Part model, mm, in its own coordinate system. Coordinates: 2 decimals unless noted, no trailing zeros. Loops run counter-clockwise (first coordinate to the right, second up) from the corner with the lowest first, then second, coordinate; pieces in that order, holes last. Notation, with made-up numbers: (-2, -29.75) -> (3, -29.75) arc R8 ccw to (3, -16.75) -> close; hole circle Ø2 at (-30, 59). An arc over 180 degrees is marked (long way). Use one line per item in the form item = value. Start each with the question number.
(1) Mould opens along Z. For faces 1 (the flat face through (0, 0, -9.525)), 2 (the flat face through (0, -4.762, 0)), 3 (the cylindrical face through (-10.349, -0.062, 1.584)) say: +Z half, -Z half, draft (parallel to the pull), parting line (faces both ways), or undercut.
(2) Band-saw the part on B-B on y = 3.5. Give the cut face in (x, z) (1 decimal), then the cut area to 3 significant figures.
(3) Drill centre lines: L1, parallel to X at y = -3, z = 0.75; L2, parallel to X at y = 1, z = -1; L3, parallel to Z at x = 1.75, y = -4.5. Where is each one in solid material? Low to high. Write a range as [from, to].
(4) Band-saw the part on A-A on z = 0. Give the cut face in (x, y) (1 decimal), then the cut area to 3 significant figures.
Autodesk Inventor part; units mm, degrees
ref_plane "YZ Plane" through (0, 0, 0) normal (1, 0, 0) x (0, 1, 0)
ref_plane "XZ Plane" through (0, 0, 0) normal (0, 1, 0) x (-1, 0, 0)
ref_plane "XY Plane" through (0, 0, 0) normal (0, 0, 1) x (1, 0, 0)
sketch "Sketch1" plane through (0, 0, 0) normal (0, 1, 0) x (-1, 0, 0)
  line L0 (-12.7, -9.525) -> (12.7, -9.525)
  line L1 (12.7, -9.525) -> (12.7, 9.525)
  line L2 (12.7, 9.525) -> (-12.7, 9.525)
  line L3 (-12.7, 9.525) -> (-12.7, -9.525)
  line L4 (-12.7, -9.525) -> (12.7, 9.525) construction
  line L5 (12.7, -9.525) -> (-12.7, 9.525) construction
  circle A0 centre (9.525, 0) radius 1.7859
  circle A1 centre (-9.525, 0) radius 1.7859
  point P0 (0, 0)
  dimension "d0" = 25.4
  dimension "d1" = 19.05
  dimension "d2" = 3.5719
  dimension "d3" = 3.5719
  dimension "d4" = 19.05
  dimension "d5" = 3.175
  dimension "d6" = 3.175
  dimension "d7" = 5.715
extrude "Extrusion1" add sketch "Sketch1" along normal mid plane 9.525
fillet "Fillet1" radius 0.3175 16 edges at (11.3109, -4.7625, 0) (11.3109, 4.7625, 0) (-7.7391, -4.7625, 0) (-7.7391, 4.7625, 0) (0, -4.7625, -9.525) (12.7, -4.7625, 0) (0, -4.7625, 9.525) (-12.7, -4.7625, 0) (12.7, 0, -9.525) (12.7, 4.7625, 0) (12.7, 0, 9.525) (0, 4.7625, 9.525) (-12.7, 0, 9.525) (-12.7, 4.7625, 0) (-12.7, 0, -9.525) (0, 4.7625, -9.525)
properties part number "enginefoot" material "Steel, Carbon"
A:
q1.face_1 = -Z half
q1.face_2 = draft
q1.face_3 = undercut
q2.outline = (-12.7, -9.2) arc R0.3 ccw to (-12.4, -9.5) -> (12.4, -9.5) arc R0.3 ccw to (12.7, -9.2) -> (12.7, 9.2) arc R0.3 ccw to (12.4, 9.5) -> (-12.4, 9.5) arc R0.3 ccw to (-12.7, 9.2) -> close; hole circle Ø3.6 at (-9.5, 0); hole circle Ø3.6 at (9.5, 0)
q2.area = 464 mm²
q3.L1 = [-12.7, -11.15], [-7.9, 7.9], [11.15, 12.7]
q3.L2 = [-12.7, -11], [-8.05, 8.05], [11, 12.7]
q3.L3 = [-9.52, 9.52]
q4.outline = (-12.7, -4.4) arc R0.3 ccw to (-12.4, -4.8) -> (-11.6, -4.8) arc R0.3 ccw to (-11.3, -4.4) -> (-11.3, 4.4) arc R0.3 ccw to (-11.6, 4.8) -> (-12.4, 4.8) arc R0.3 ccw to (-12.7, 4.4) -> close; (-7.7, -4.4) arc R0.3 ccw to (-7.4, -4.8) -> (7.4, -4.8) arc R0.3 ccw to (7.7, -4.4) -> (7.7, 4.4) arc R0.3 ccw to (7.4, 4.8) -> (-7.4, 4.8) arc R0.3 ccw to (-7.7, 4.4) -> close; (11.3, -4.4) arc R0.3 ccw to (11.6, -4.8) -> (12.4, -4.8) arc R0.3 ccw to (12.7, -4.4) -> (12.7, 4.4) arc R0.3 ccw to (12.4, 4.8) -> (11.6, 4.8) arc R0.3 ccw to (11.3, 4.4) -> close
q4.area = 174 mm²
